Read the model definition and answer for the solid it produces. Units are mm, in the model's axes. A direction names the side the tool comes from. Coordinates: 2 decimals unless noted, no trailing zeros. Order: outer loops, then holes, each group sorted by start corner. A loop starts at its lowest first (then second) coordinate and runs counter-clockwise, first axis right, second up. Notation, with made-up numbers: M 17,85 L 70,85 A11 cw 70,92 Z; hole C 61.5,-38 d2. An arc over 180 degrees is marked long. Write each question's results on one line, items separated by ' | '.
```python
from build123d import *

# Parameters (mm, degrees)
EXTRUDE_1_DEPTH     = 2
SKETCH_2_W          = 6
SKETCH_2_H          = 2
EXTRUDE_2_DEPTH     = 3.5
FILLET_1_R          = 3
SKETCH_3_R          = 1
CUT_EXTRUDE_1_DEPTH = 5
CUT_EXTRUDE_1_DRAFT = -2
SKETCH_4_R          = 1
CUT_EXTRUDE_2_DEPTH = 5
CUT_EXTRUDE_2_DRAFT = -2
SKETCH_6_W          = 3.6
SKETCH_6_H          = 2
EXTRUDE_3_DEPTH     = 3
CHAMFER_1_SIZE      = 3
SKETCH_7_R          = 0.75
EXTRUDE_4_DEPTH     = 3
CUT_EXTRUDE_3_REACH = 30.118
SKETCH_8_W          = 3
SKETCH_8_H          = 1.5
FILLET_2_R          = 0.75


# Some blends are built 0.0001 mm under size
with BuildPart() as part:
    # 草图1 → 凸台-拉伸1 (new body)
    with BuildSketch(Plane.XY):
        with BuildLine():
            Line((-11.942385676, 3.311338927), (-11.942385676, -22.488661073))
            Line((-11.942385676, -22.488661073), (14.057614324, -22.488661073))
            ThreePointArc((14.057614324, -22.488661073), (15.401117208, -21.932163957), (15.957614324, -20.588661073))
            Line((15.957614324, -20.588661073), (15.957614324, 1.411338927))
            ThreePointArc((15.957614324, 1.411338927), (15.401117208, 2.754841811), (14.057614324, 3.311338927))
            Line((14.057614324, 3.311338927), (-11.942385676, 3.311338927))
        make_face()
    extrude(amount=-EXTRUDE_1_DEPTH)

    # 草图2 → 凸台-拉伸2 (add)
    with BuildSketch(Plane(origin=(0, 0, -2), x_dir=(-1, 0, 0), z_dir=(0, 0, -1))):
        with Locations((-8.857614324, -21.488661073)):
            Rectangle(SKETCH_2_W, SKETCH_2_H)
        with Locations((-8.857614324, 2.311338927)):
            Rectangle(SKETCH_2_W, SKETCH_2_H)
    extrude(amount=EXTRUDE_2_DEPTH)

    # 圆角1
    fillet_1_edges = [part.edges().sort_by_distance(p)[0] for p in [
        (11.857614324, 2.311338927, -5.5),
        (5.857614324, 2.311338927, -5.5),
        (11.857614324, -21.488661073, -5.5),
        (5.857614324, -21.488661073, -5.5),
    ]]
    fillet(fillet_1_edges, radius=FILLET_1_R - 0.0001)  # a hair under: the kernel refuses the full size


with BuildPart() as cut_extrude_1_tool:
    # 草图3 → 切除-拉伸1 (with draft: the straight prism first)
    with BuildSketch(Plane.XZ.offset(22.488661073)):
        with Locations((8.874069652, -2.5)):
            Circle(SKETCH_3_R)
    extrude(amount=-CUT_EXTRUDE_1_DEPTH)
    # 切除-拉伸1: the draft: its side faces are tilted about the plane it starts from
    cut_extrude_1_sides = [cut_extrude_1_tool.faces().sort_by_distance(p)[0] for p in [
        (7.874069652, -19.988661073, -2.5),
    ]]
    draft(cut_extrude_1_sides, Plane.XZ.offset(22.488661073), CUT_EXTRUDE_1_DRAFT)


with BuildPart() as part_1:
    add(part.part)

    # 切除-拉伸1: cut by cut_extrude_1_tool
    add(cut_extrude_1_tool.part, mode=Mode.SUBTRACT)


with BuildPart() as cut_extrude_2_tool:
    # 草图4 → 切除-拉伸2 (with draft: the straight prism first)
    with BuildSketch(Plane(origin=(0, 3.311338927, 0), x_dir=(1, 0, 0), z_dir=(0, 1, 0))):
        with Locations((8.874069652, 2.5)):
            Circle(SKETCH_4_R)
    extrude(amount=-CUT_EXTRUDE_2_DEPTH)
    # 切除-拉伸2: the draft: its side faces are tilted about the plane it starts from
    cut_extrude_2_sides = [cut_extrude_2_tool.faces().sort_by_distance(p)[0] for p in [
        (7.874069652, 0.811338927, -2.5),
    ]]
    draft(cut_extrude_2_sides, Plane(origin=(0, 3.311338927, 0), x_dir=(1, 0, 0), z_dir=(0, 1, 0)), CUT_EXTRUDE_2_DRAFT)


with BuildPart() as part_2:
    add(part_1.part)

    # 切除-拉伸2: cut by cut_extrude_2_tool
    add(cut_extrude_2_tool.part, mode=Mode.SUBTRACT)

    # 草图6 → 凸台-拉伸3 (add)
    with BuildSketch(Plane.XY):
        with Locations((-13.742385676, -1.688661073)):
            Rectangle(SKETCH_6_W, SKETCH_6_H)
        with Locations((-13.742385676, -17.488661073)):
            Rectangle(SKETCH_6_W, SKETCH_6_H)
    extrude(amount=-EXTRUDE_3_DEPTH)

    # 倒角1
    # the kernel refuses this chamfer: 3 mm, written as the material it adds along each edge
    with BuildSketch(Plane(origin=(-11.942385676, -16.488661073, -2), x_dir=(0.9996219169112969, 0, 0.027495876610586355), z_dir=(0, -1, 0))) as chamfer_1_piece_1_section:
        Polygon((CHAMFER_1_SIZE * 0.999621916911, -CHAMFER_1_SIZE * 0.0274958766106), (-CHAMFER_1_SIZE * 0.0274958766106, -CHAMFER_1_SIZE * 0.999621916911), (0, 0), align=None)
    chamfer_1_piece_1 = extrude(amount=2, mode=Mode.PRIVATE)
    chamfer_1_piece_1 = split(chamfer_1_piece_1, bisect_by=Plane(origin=(-10.675719009, -17.488661073, -3), z_dir=(0, 0, 1)), keep=Keep.TOP, mode=Mode.PRIVATE)
    add(chamfer_1_piece_1)
    with BuildSketch(Plane(origin=(-11.942385676, -0.688661073, -2), x_dir=(0.9996219169112969, 0, 0.027495876610586355), z_dir=(0, -1, 0))) as chamfer_1_piece_2_section:
        Polygon((CHAMFER_1_SIZE * 0.999621916911, -CHAMFER_1_SIZE * 0.0274958766106), (-CHAMFER_1_SIZE * 0.0274958766106, -CHAMFER_1_SIZE * 0.999621916911), (0, 0), align=None)
    chamfer_1_piece_2 = extrude(amount=2, mode=Mode.PRIVATE)
    chamfer_1_piece_2 = split(chamfer_1_piece_2, bisect_by=Plane(origin=(-10.675719009, -1.688661073, -3), z_dir=(0, 0, 1)), keep=Keep.TOP, mode=Mode.PRIVATE)
    add(chamfer_1_piece_2)

    # 草图7 → 凸台-拉伸4 (add)
    with BuildSketch(Plane.XY):
        with Locations((-14.792385676, -0.688661073)):
            Circle(SKETCH_7_R)
        with Locations((-14.792385676, -18.488661073)):
            Circle(SKETCH_7_R)
    extrude(amount=-EXTRUDE_4_DEPTH)

    # 草图8 → 切除-拉伸3 (cut, up to next)
    with BuildSketch(Plane.XY, mode=Mode.PRIVATE) as cut_extrude_3_sk1:
        with Locations((-10.442385676, -3.438661073)):
            Rectangle(SKETCH_8_W, SKETCH_8_H)
    cut_extrude_3_tool1 = extrude(cut_extrude_3_sk1.sketch, amount=-CUT_EXTRUDE_3_REACH, mode=Mode.PRIVATE) & part_2.part
    # 草图8 → 切除-拉伸3 (cut, up to next)
    with BuildSketch(Plane.XY, mode=Mode.PRIVATE) as cut_extrude_3_sk2:
        with Locations((-10.442385676, 0.061338927)):
            Rectangle(SKETCH_8_W, SKETCH_8_H)
    cut_extrude_3_tool2 = extrude(cut_extrude_3_sk2.sketch, amount=-CUT_EXTRUDE_3_REACH, mode=Mode.PRIVATE) & part_2.part
    # 草图8 → 切除-拉伸3 (cut, up to next)
    with BuildSketch(Plane.XY, mode=Mode.PRIVATE) as cut_extrude_3_sk3:
        with Locations((-10.442385676, -15.738661073)):
            Rectangle(SKETCH_8_W, SKETCH_8_H)
    cut_extrude_3_tool3 = extrude(cut_extrude_3_sk3.sketch, amount=-CUT_EXTRUDE_3_REACH, mode=Mode.PRIVATE) & part_2.part
    # 草图8 → 切除-拉伸3 (cut, up to next)
    with BuildSketch(Plane.XY, mode=Mode.PRIVATE) as cut_extrude_3_sk4:
        with Locations((-10.442385676, -19.238661073)):
            Rectangle(SKETCH_8_W, SKETCH_8_H)
    cut_extrude_3_tool4 = extrude(cut_extrude_3_sk4.sketch, amount=-CUT_EXTRUDE_3_REACH, mode=Mode.PRIVATE) & part_2.part
    add(cut_extrude_3_tool1.solids().sort_by_distance((-10.442386, -3.438661, 0))[0], mode=Mode.SUBTRACT)
    add(cut_extrude_3_tool2.solids().sort_by_distance((-10.442386, 0.061339, 0))[0], mode=Mode.SUBTRACT)
    add(cut_extrude_3_tool3.solids().sort_by_distance((-10.442386, -15.738661, 0))[0], mode=Mode.SUBTRACT)
    add(cut_extrude_3_tool4.solids().sort_by_distance((-10.442386, -19.238661, 0))[0], mode=Mode.SUBTRACT)

    # 圆角2
    fillet_2_edges = [part_2.edges().sort_by_distance(p)[0] for p in [
        (-8.942385676, -2.688661073, -1),
        (-8.942385676, 0.811338927, -1),
        (-8.942385676, -18.488661073, -1),
        (-8.942385676, -14.988661073, -1),
        (-8.942385676, -19.988661073, -1),
        (-8.942385676, -16.488661073, -1),
        (-8.942385676, -4.188661073, -1),
        (-8.942385676, -0.688661073, -1),
    ]]
    fillet(fillet_2_edges, radius=FILLET_2_R - 0.0001)  # a hair under: the kernel refuses the full size


solid = part_2.part
```
(1) The part is cut by section A-A, the plane z = -4.7. Write down the section's boundary in (x, y), then the cut area to 3 significant figures.
Conclusion:
outline: M 6.82,-22.49 L 10.9,-22.49 L 10.9,-20.49 L 6.82,-20.49 Z; M 6.82,1.31 L 10.9,1.31 L 10.9,3.31 L 6.82,3.31 Z | area: 16.3 mm²
(2) Straight lines are drawn through the part: line 1 (Y direction, x = 11, z = -3.2); line 2 (Z direction, x = 5.5, y = 0.5); line 3 (X direction, y = -4.75, z = -0.4). For each, find the intervals that lie inside material, in ascending order.
Conclusion:
line 1: -22.49 to -20.49, 1.31 to 3.31 | line 2: -2 to 0 | line 3: -11.94 to 15.96
(3) For faces 1 (the flat face through (9, -20.489, -4)), 2 (the flat face through (-11, -4.189, -1)), 3 (the flat face through (-11.942, -21, -1)), determine the directions among +Z, -Z, +X, -X, +Y, -Y from which every point of the face is accessible in a straight line to the end or side of a thin tool.
Conclusion:
face 1: -Z, +X, -X | face 2: +Z, -Z, -X | face 3: +Z, -Z, -X, -Y
(4) The mould has two halves that part along Z. Classify faces 4 (the flat face through (-9.435, -1.664, -2.493)), 5 (the flat face through (4, 3.311, -1)), 6 (the conical face through (8.753, -20.579, -1.575)): pulls with the +Z half, pulls with the -Z half, needs draft (parallel to the pull), parting line crosses it, or undercut.
Conclusion:
face 4: pulls with the -Z half | face 5: needs draft | face 6: undercut
(5) The part is cut by section B-B, the plane x = 2.5. Write down the section's boundary in (y, z), then the cut area to 3 significant figures.
Conclusion:
outline: M -22.49,-2 L 3.31,-2 L 3.31,0 L -22.49,0 Z | area: 51.6 mm²
(6) Given pin 1 (3 mm diameter, centred on x = -12, y = -17.5, fed in from -Z); pin 2 (2 mm diameter, centred on y = -7.5, z = -2.5, fed in from -X); pin 3 (1.5 mm diameter, centred on x = 9, z = -3, fed in from +Y); pin 4 (0.6 mm diameter, centred on y = 2.5, z = -2.5, fed in from -X), each flat-ended and moving along its own axis, determine where each tip first touches the part or whether it passes through.
Conclusion:
pin 1: z = -3 | pin 2: x = -11.94 | pin 3: y = 3.31 | pin 4: x = 5.86
(7) The part is cut by section C-C, the plane y = -6.25. Write down the section's boundary in (x, z), then the cut area to 3 significant figures.
Conclusion:
outline: M -11.94,-2 L 15.96,-2 L 15.96,0 L -11.94,0 Z | area: 55.8 mm²
